Design review of the part built by this model. Coordinates are the model's own, in mm. Face numbers are marked on the shaded views. A direction names the side the tool comes from. Coordinates: 2 decimals unless noted, no trailing zeros. Write each loop counter-clockwise with the first axis right and the second up, starting at its lowest first coordinate (ties: lowest second). Pieces come first, ordered by that corner, then holes.
Q1. Take a section at C-C, the plane y = 0.5. State how many separate pieces and enclosed holes the cut face has, plus the area to 3 significant figures.
Q2. For pin 1 Ø7 at (x, z) = (15, 6) entering from -Y; pin 2 Ø1.3 at (x, z) = (3, 9) entering from -Y, all flat-tipped, find the tip position at first contact; note any pin that passes through.
Q3. For the marked faces 4, 5 and 6, list the 3-axis set-ups (+Z, -Z, +X, -X, +Y, -Y) from which the entire face can be reached by the end or side of a thin tool; tool diameter is ignored.
Q4. Take a section at A-A, the plane z = 6. Write out the cut boundary in (x, y).
Q5. For L1, parallel to Z at x = 9.2, y = 0.6; L2, parallel to X at y = 1.85, z = 6; L3, parallel to Z at x = 17.75, y = 1.2, list the stretches that pass through material, from the lowest coordinate up.
Q6. Take a section at D-D, the plane x = 10.25. Write out the cut boundary in (y, z).
Q7. The part is to be moulded in two halves that separate along X. For the marked faces 1, 2 and 3, say which applies: released by +X, released by -X, zero draft, split by the parting line, or undercut.
Q8. Take a section at B-B, the plane z = 9. Write out the cut boundary in (x, y), plus the area to 3 significant figures.
from build123d import *

# Parameters (mm, degrees)
SKETCH_1_W          = 20
SKETCH_1_H          = 12
SKETCH_1_R          = 1.6
SKETCH_1_R_2        = 2.6
SKETCH_1_R_3        = 1
EXTRUDE_1_DEPTH     = 2.5
EXTRUDE_START       = 1.5
SKETCH_1_5_R        = 1.6
SKETCH_1_5_R_2      = 0.75
EXTRUDE_2_DEPTH     = 1
SKETCH_3_R          = 0.7
SKETCH_3_R_2        = 0.35
CUT_EXTRUDE_1_DEPTH = 24.457408211
SKETCH_3_3_R        = 1
CUT_EXTRUDE_2_DEPTH = 1.5


with BuildPart() as part:
    # 草图1 → 凸台-拉伸1 (new body)
    with BuildSketch(Plane(origin=(0, 0, 0), x_dir=(1, 0, 0), z_dir=(0, 1, 0))):
        with Locations((10, -6)):
            Rectangle(SKETCH_1_W, SKETCH_1_H)
        with Locations(Location((9.2, -6, 0), (0, 0, 270))):
            Circle(SKETCH_1_R, mode=Mode.SUBTRACT)
        with Locations(Location((15, -6, 0), (0, 0, 270))):
            Circle(SKETCH_1_R_2, mode=Mode.SUBTRACT)
        with Locations(Location((5, -6, 0), (0, 0, 270))):
            Circle(SKETCH_1_R_3, mode=Mode.SUBTRACT)
    extrude(amount=EXTRUDE_1_DEPTH)

    # 草图1<5> → 凸台-拉伸2 (add)
    with BuildSketch(Plane(origin=(0, 0, 0), x_dir=(1, 0, 0), z_dir=(0, 1, 0)).offset(EXTRUDE_START)):
        with Locations(Location((9.2, -6, 0), (0, 0, 90))):
            Circle(SKETCH_1_5_R)
        with Locations(Location((9.2, -6, 0), (0, 0, 90))):
            Circle(SKETCH_1_5_R_2, mode=Mode.SUBTRACT)
    extrude(amount=EXTRUDE_2_DEPTH)

    # 草图3 → 切除-拉伸1 (cut, through all)
    with BuildSketch(Plane(origin=(0, 2.5, 0), x_dir=(1, 0, 0), z_dir=(0, 1, 0))):
        with Locations(Location((3, -9, 0), (0, 0, 270))):
            Circle(SKETCH_3_R)
        with Locations(Location((6, -2, 0), (0, 0, 270))):
            Circle(SKETCH_3_R)
        with Locations(Location((17, -1.5, 0), (0, 0, 270))):
            Circle(SKETCH_3_R)
        with Locations(Location((17, -10.5, 0), (0, 0, 270))):
            Circle(SKETCH_3_R)
        with Locations(Location((3, -3, 0), (0, 0, 270))):
            Circle(SKETCH_3_R_2)
        with Locations(Location((6, -10, 0), (0, 0, 270))):
            Circle(SKETCH_3_R_2)
        with Locations(Location((13, -10, 0), (0, 0, 270))):
            Circle(SKETCH_3_R_2)
        with Locations(Location((13, -2, 0), (0, 0, 270))):
            Circle(SKETCH_3_R_2)
    extrude(amount=-CUT_EXTRUDE_1_DEPTH, mode=Mode.SUBTRACT)

    # 草图3<3> → 切除-拉伸2 (cut)
    with BuildSketch(Plane(origin=(0, 2.5, 0), x_dir=(1, 0, 0), z_dir=(0, 1, 0))):
        with Locations(Location((6, -2, 0), (0, 0, 270))):
            Circle(SKETCH_3_3_R)
        with Locations(Location((3, -9, 0), (0, 0, 270))):
            Circle(SKETCH_3_3_R)
        with Locations(Location((17, -1.5, 0), (0, 0, 270))):
            Circle(SKETCH_3_3_R)
        with Locations(Location((17, -10.5, 0), (0, 0, 270))):
            Circle(SKETCH_3_3_R)
    extrude(amount=-CUT_EXTRUDE_2_DEPTH, mode=Mode.SUBTRACT)


solid = part.part
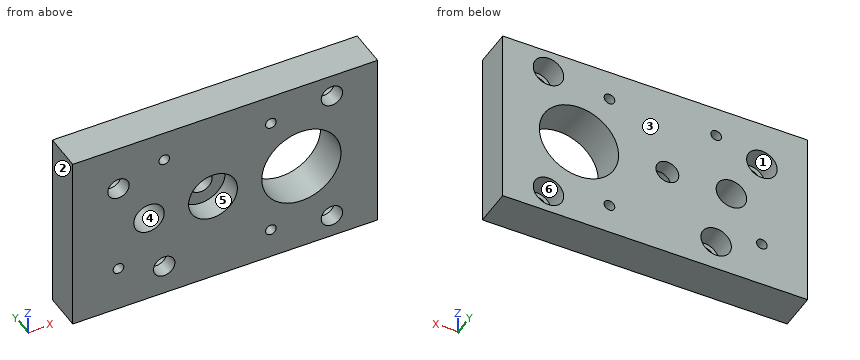
Responses:
1. separate pieces: 1
1. enclosed holes: 11
1. area: 200 mm2
2. pin 1: stops at y = 0
2. pin 2: passes through
3. face 4: +Y, -Y
3. face 5: -Y
3. face 6: +Y
4. outline: (0, 0) - (4, 0) - (4, 2.5) - (0, 2.5) - close; (6, 0) - (7.6, 0) - (7.6, 1.5) - (8.45, 1.5) - (8.45, 2.5) - (6, 2.5) - close; (9.95, 1.5) - (10.8, 1.5) - (10.8, 0) - (12.4, 0) - (12.4, 2.5) - (9.95, 2.5) - close; (17.6, 0) - (20, 0) - (20, 2.5) - (17.6, 2.5) - close
5. L1: z = 0 to 4.4, 7.6 to 12
5. L2: x = 0 to 4, 6 to 8.45, 9.95 to 12.4, 17.6 to 20
5. L3: z = 0 to 0.84, 2.16 to 9.84, 11.16 to 12
6. outline: (0, 0) - (2.5, 0) - (2.5, 12) - (0, 12) - (0, 7.21) - (1.5, 7.21) - (1.5, 4.79) - (0, 4.79) - close
7. face 1: undercut
7. face 2: released by -X
7. face 3: zero draft
8. outline: (0, 0) - (2.3, 0) - (2.3, 1) - (2, 1) - (2, 2.5) - (0, 2.5) - close; (3.7, 0) - (20, 0) - (20, 2.5) - (4, 2.5) - (4, 1) - (3.7, 1) - close
8. area: 45.6 mm2
